For this review, take the finished solid that the model builds, in its own axes (mm). Face numbers are marked on the shaded views. Round coordinates to 2 decimals unless told otherwise and drop trailing zeros. Order: outer loops, then holes, each group sorted by start corner. A loop starts at its lowest first (then second) coordinate and runs counter-clockwise, first axis right, second up.
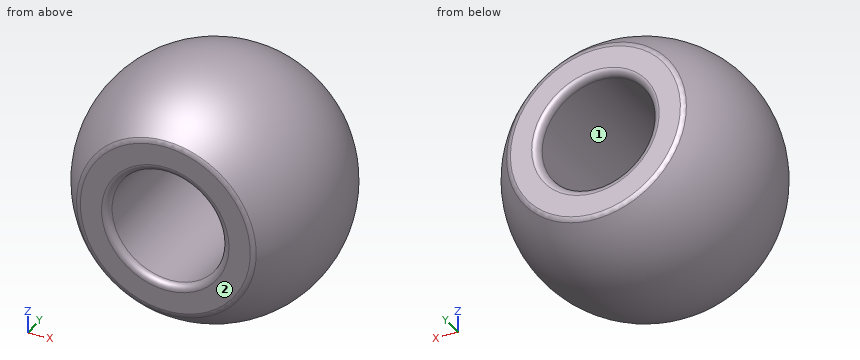
```python
from build123d import *

# Parameters (mm, degrees)
FILLET1_R = 0.3


with BuildPart() as part:
    # Sketch1 → Revolve1 (revolve)
    with BuildSketch(Plane.XY):
        with BuildLine():
            Line((3.854610875, 4), (2.5, 4))
            Line((2.5, 4), (2.5, -4))
            Line((2.5, -4), (3.854610875, -4))
            ThreePointArc((3.854610875, -4), (5.555, 0), (3.854610875, 4))
        make_face()
    revolve(axis=Axis((0, 4, 0), (0, -1, 0)))

    # Fillet1
    fillet1_edges = [part.edges().sort_by_distance(p)[0] for p in [
        (-3.854610875, -4, 0),
        (-2.5, -4, 0),
        (-2.5, 4, 0),
        (-3.854610875, 4, 0),
    ]]
    fillet(fillet1_edges, radius=FILLET1_R)


solid = part.part
```
Q1. Take a section at B-B, the plane z = 4.5. State the section outline as (x, y) points.
Q2. Wall thickness on line 1 (X direction, y = 1.5, z = -1.25); line 2 (Z direction, x = -2.25, y = 3.25); line 3 (Z direction, x = 0, y = -0.5): over which ranges is each line inside the solid? List them lowest first.
Q3. Take a section at D-D, the plane y = -3.5. State the section outline as (x, z) points.
Q4. Clearance check with flat-ended pins moving along their axes: pin 1 (4 mm diameter, centred on y = -2.5, z = 3, fed in from +X); pin 2 (4 mm diameter, centred on x = 1.5, y = -1.5, fed in from -Z); pin 3 (2 mm diameter, centred on x = 0.5, y = 3, fed in from +Z). State where each tip first meets the part, or that it passes through.
Q5. Take a section at A-A, the plane y = 1. State the section outline as (x, z) points.
Q6. Mouldability with a two-part tool opening along Z and no side actions: class the marked faces 1 and 2 as +Z half, -Z half, draft (parallel to the pull), parting line (faces both ways), or undercut.
Working result:
1. outline: circle Ø6.51 at (0, 0)
2. line 1: x = -5.2 to -2.17, 2.17 to 5.2
2. line 2: z = -3.9 to -1.09, 1.09 to 3.9
2. line 3: z = -5.53 to -2.5, 2.5 to 5.53
3. outline: circle Ø8.63 at (0, 0); hole circle Ø5 at (0, 0)
4. pin 1: stops at x = 5.22
4. pin 2: stops at z = -5.55
4. pin 3: stops at z = 5.17
5. outline: circle Ø10.93 at (0, 0); hole circle Ø5 at (0, 0)
6. face 1: undercut
6. face 2: draft
